```python
from build123d import *

# Parameters (mm, degrees)
BOSS_EXTRUDE1_DEPTH = 2
FILLET1_R           = 5
SKETCH2_R           = 4.25
CUT_EXTRUDE1_DEPTH  = 10
SKETCH3_W           = 53.20846293
SKETCH3_H           = 69
BOSS_EXTRUDE2_DEPTH = 2
FILLET2_R           = 3


with BuildPart() as part:
    # Sketch1 → Boss-Extrude1 (new body)
    with BuildSketch(Plane.XY):
        with BuildLine():
            Line((-27.5, 15.515231625), (-27.5, 21.501022606))
            Line((-27.5, 21.501022606), (25.5, 16.795650425))
            Line((25.5, 16.795650425), (25.5, -35.408879242))
            Line((25.5, -35.408879242), (11.603178078, -34.175110954))
            ThreePointArc((11.603178078, -34.175110954), (5.026609694, -30.872744893), (2.490629392, -23.964367571))
            ThreePointArc((2.490629392, -23.964367571), (-3.555183787, -5.141257472), (-20, 5.83277326))
            ThreePointArc((-20, 5.83277326), (-25.40569415, 9.391507269), (-27.5, 15.515231625))
        make_face()
    extrude(amount=BOSS_EXTRUDE1_DEPTH)

    # Fillet1
    fillet1_edges = [part.edges().sort_by_distance(p)[0] for p in [
        (25.5, -35.408879242, 1),
    ]]
    fillet(fillet1_edges, radius=FILLET1_R)

    # Sketch2 → Cut-Extrude1 (cut)
    with BuildSketch(Plane.XY.offset(2)):
        with Locations((17.5, -26.667168282)):
            Circle(SKETCH2_R)
    extrude(amount=-CUT_EXTRUDE1_DEPTH, mode=Mode.SUBTRACT)


with BuildPart() as body_2:
    # Mirror3: mirrored copy
    add(part.part.mirror(Plane(origin=(0, 0, -32.5), x_dir=(1, 0, 0), z_dir=(0, 0, -1))))


with BuildPart() as part_1:
    add(part.part)

    add(body_2.part)  # Boss-Extrude2 merges body 2
    # Sketch3 → Boss-Extrude2 (add)
    with BuildSketch(Plane(origin=(1.678885973, 18.910503392, 0), x_dir=(0.9960821471166026, -0.08843277783479815, 0), z_dir=(0.08843277783479815, 0.9960821471166027, 0))):
        with Locations((-2.689422736, 32.5)):
            Rectangle(SKETCH3_W, SKETCH3_H)
    extrude(amount=BOSS_EXTRUDE2_DEPTH)

    # Fillet2
    fillet2_edges = [part_1.edges().sort_by_distance(p)[0] for p in [
        (-0.823134444, 21.140500809, 2),
        (-0.823134444, 21.140500809, -67),
    ]]
    fillet(fillet2_edges, radius=FILLET2_R)


solid = part_1.part
```
Work out the finished part from the listing and answer in its coordinate system (mm). A direction names the side the tool comes from. Give positions to 0.01 mm unless a question says otherwise; leave off trailing zeros. Write each loop counter-clockwise with the first axis right and the second up, starting at its lowest first coordinate (ties: lowest second). Pieces come first, ordered by that corner, then holes. Notation, with made-up numbers: (10.5, -30) - (38.5, -30) arc R21 ccw to (38.5, 0) - close; hole circle Ø1 at (-18, 29.25). An arc over 180 degrees is marked (long way). Use one line per item in the form item = value.
1. Each of these flat-tipped pins is pushed along its axis until it touches: pin 1 Ø12 at (x, y) = (-4.5, -28.5) entering from +Z; pin 2 Ø3 at (x, z) = (16, -52) entering from +Y; pin 3 Ø8 at (x, z) = (16.5, -12.5) entering from -Y; pin 4 Ø12 at (x, z) = (-3.5, -12) entering from -Y. Where does it stop, or does it pass through?
Filled in:
pin_1 = through
pin_2 = 19.78
pin_3 = 17.24
pin_4 = 18.84
2. A cutting plane is placed at D-D (x = 17.5). State how many separate pieces and enclosed holes the cut face has, and give its area (3 significant figures).
Filled in:
separate_pieces = 3
enclosed_holes = 0
area = 309 mm^2
3. A cutting plane is placed at C-C (y = -20.5). Write down the section's boundary in (x, z).
Filled in:
outline = (2.38, -67) - (25.5, -67) - (25.5, -65) - (2.38, -65) - close; (2.38, 0) - (25.5, 0) - (25.5, 2) - (2.38, 2) - close
4. For faces 5 (the face through (5, -3, 2)), 6 (the face through (25.5, -6, 1)), determine the directions among +Z, -Z, +X, -X, +Y, -Y from which every point of the face is accessible in a straight line to the end or side of a thin tool.
Filled in:
face_5 = +Z, +X, -X, +Y, -Y
face_6 = +Z, -Z, +X, -Y
5. Consider L1, parallel to Z at x = 6, y = -9; L2, parallel to Z at x = -1.5, y = 19; L3, parallel to Y at x = 17.5, z = -65.9. Determine where each line is inside the solid, lowest interval first.
Filled in:
L1 = -67 to -65, 0 to 2
L2 = -66.89 to -65, 0 to 1.89
L3 = -34.7 to -30.92, -22.42 to 18.83
6. Determine the mould class of faces 1 (the face through (5, 0, -65)), 2 (the face through (25.587, 17.778, -32.019)), 3 (the face through (-25.35, 9.32, 0.99)), 4 (the face through (14.127, -29.253, 1.014)) for opening direction X: released by +X, released by -X, zero draft, split by the parting line, or undercut.
Filled in:
face_1 = zero draft
face_2 = released by +X
face_3 = released by -X
face_4 = undercut
7. A cutting plane is placed at A-A (y = -12). Write down the section's boundary in (x, z).
Filled in:
outline = (0.33, -67) - (25.5, -67) - (25.5, -65) - (0.33, -65) - close; (0.33, 0) - (25.5, 0) - (25.5, 2) - (0.33, 2) - close
8. A cutting plane is placed at B-B (z = -4). Write down the section's boundary in (x, y), and give its area (3 significant figures).
Filled in:
outline = (-27.5, 21.5) - (25.5, 16.8) - (25.68, 18.79) - (-27.32, 23.49) - close
area = 106 mm^2
